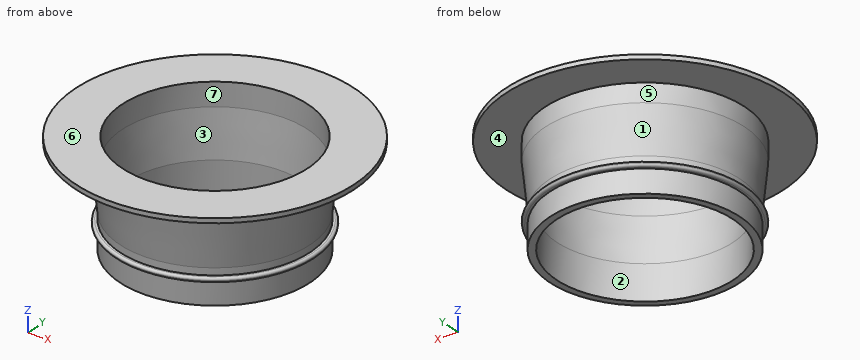
from build123d import *

# Parameters (mm, degrees)
F2_R     = 76.2
F2_R_2   = 54.6292916326
F2_R_3   = 52.1095022643
F3_DEPTH = 2.54
F4_R     = 1.26999


# Not quite as in the source:
# - a fillet or chamfer is up to 0.001 mm smaller than in the source, because OpenCascade refuses the exact size


with BuildPart() as f1:
    # F0 (on Right) → F1 (revolve)
    with BuildSketch(Plane.YZ):
        Polygon((-48.2407083674, -19.05), (-48.2407083674, 0), (-50.8, 25.4), (-50.8, 38.1), (-54.6292916326, 38.1), (-54.6292916326, 25.4), (-52.07, 0), (-52.07, -3.81), (-54.61, -3.81), (-54.61, -6.35), (-52.07, -6.35), (-52.07, -19.05), align=None)
    revolve(axis=Axis((0, 0, 19.0012101084), (0, 0, -1)))

    # F2 (on face) → F3 (join)
    with BuildSketch(Plane.XY.offset(38.1)):
        Circle(F2_R)
        Circle(F2_R_2, mode=Mode.SUBTRACT)
        Circle(F2_R_2)
        Circle(F2_R_3, mode=Mode.SUBTRACT)
    extrude(amount=-F3_DEPTH)

    # F4 (radius 1.27 in the source; OpenCascade refuses exactly that, so slightly less here)
    f4_edges = [f1.edges().sort_by_distance(p)[0] for p in [
        (0, 54.61, -3.81),
        (0, 54.61, -6.35),
    ]]
    fillet(f4_edges, radius=F4_R)


solid = f1.part
The model under review builds one solid part; all positions refer to its coordinate system, in mm. Face numbers are marked on the shaded views. A direction names the side the tool comes from. Round coordinates to 2 decimals unless told otherwise and drop trailing zeros. Order: outer loops, then holes, each group sorted by start corner. A loop starts at its lowest first (then second) coordinate and runs counter-clockwise, first axis right, second up. Notation, with made-up numbers: (42, 49) -> (70, 49) arc R26 cw to (70, 73) -> close; hole circle Ø7 at (38, 48). An arc over 180 degrees is marked (long way). Use CSV: the item, a comma, the result in double quotes. Start each with the question number.
(1) Wall thickness on probe 1 along Y at (x, z) = (-0.5, -16); probe 2 along Y at (x, z) = (0, 31): over which ranges is each line inside the solid? List them lowest first. Write a range as from..to.
(2) Consider section D-D on z = 2. Write out the cut boundary in (x, y), and give its area (3 significant figures).
(3) Tool access review of the marked faces 5, 6 and 7: name each direction out of +Z, -Z, +X, -X, +Y, -Y from which nothing blocks a thin tool from reaching the whole face with its end or side.
(4) Mouldability with a two-part tool opening along X and no side actions: class the marked faces 1, 2, 3 and 4 as pulls with the +X half, pulls with the -X half, needs draft (parallel to the pull), parting line crosses it, or undercut.
(5) Consider section C-C on z = -12. Write out the cut boundary in (x, y).
(6) Insertion check: pin 1 (8 mm diameter, centred on x = 55, y = -18.5, fed in from -Z); pin 2 (8 mm diameter, centred on x = -46.5, z = 31.5, fed in from +Y); pin 3 (3 mm diameter, centred on y = -14, z = 32, fed in from +X). Each pin has a flat end and moves straight along its axis. Give the tip position at first contact, or say it passes through.
Responses:
1,probe 1,"-52.07..-48.24, 48.24..52.07"
1,probe 2,"-54.63..-50.8, 50.8..54.63"
2,outline,"circle Ø104.54 at (0, 0); hole circle Ø96.88 at (0, 0)"
2,area,"1,210 mm²"
3,face 5,"-Z"
3,face 6,"+Z, +X, -X, +Y, -Y"
3,face 7,"+Z"
4,face 1,"parting line crosses it"
4,face 2,"undercut"
4,face 3,"undercut"
4,face 4,"needs draft"
5,outline,"circle Ø104.14 at (0, 0); hole circle Ø96.48 at (0, 0)"
6,pin 1,"z = -6.15"
6,pin 2,"y = 34.32"
6,pin 3,"x = 53.18"
